Design review of the part built by this model. Coordinates are the model's own, in mm. A direction names the side the tool comes from. Coordinates: 2 decimals unless noted, no trailing zeros. Order: outer loops, then holes, each group sorted by start corner. A loop starts at its lowest first (then second) coordinate and runs counter-clockwise, first axis right, second up. Notation, with made-up numbers: (79.25, -28.75) - (86.25, -28.75) arc R20 cw to (86.25, -6.75) - close; hole circle Ø8 at (81, 15.5). An arc over 180 degrees is marked (long way). Write each question's results on one line, items separated by ' | '. Start each with the question number.
```python
from build123d import *

# Parameters (mm, degrees)
BOSS_EXTRUDE4_DEPTH = 5
SKETCH6_W           = 70
SKETCH6_H           = 70
BOSS_EXTRUDE5_DEPTH = 20
SKETCH8_R           = 3
CUT_EXTRUDE1_DEPTH  = 2
FILLET1_R           = 10
SKETCH9_W           = 24
SKETCH9_H           = 2.25
CUT_EXTRUDE2_DEPTH  = 15
SKETCH10_W          = 11.25
SKETCH10_H          = 1
CUT_EXTRUDE3_DEPTH  = 10
CHAMFER1_SIZE       = 1


with BuildPart() as part:
    # Sketch5 → Boss-Extrude4 (new body)
    with BuildSketch(Plane(origin=(0, 0, 0), x_dir=(1, 0, 0), z_dir=(0, 1, 0))):
        with BuildLine():
            Line((-22.5, -32.5), (22.5, -32.5))
            ThreePointArc((22.5, -32.5), (29.571067812, -29.571067812), (32.5, -22.5))
            Line((32.5, -22.5), (32.5, 22.5))
            ThreePointArc((32.5, 22.5), (29.571067812, 29.571067812), (22.5, 32.5))
            Line((22.5, 32.5), (-22.5, 32.5))
            ThreePointArc((-22.5, 32.5), (-29.571067812, 29.571067812), (-32.5, 22.5))
            Line((-32.5, 22.5), (-32.5, -22.5))
            ThreePointArc((-32.5, -22.5), (-29.571067812, -29.571067812), (-22.5, -32.5))
        make_face()
    extrude(amount=BOSS_EXTRUDE4_DEPTH)

    # Sketch6 → Boss-Extrude5 (add)
    with BuildSketch(Plane(origin=(0, 5, 0), x_dir=(1, 0, 0), z_dir=(0, 1, 0))):
        Rectangle(SKETCH6_W, SKETCH6_H)
    extrude(amount=BOSS_EXTRUDE5_DEPTH)

    # Sketch8 → Cut-Extrude1 (cut)
    with BuildSketch(Plane.XZ):
        with Locations(Location((26.037533906, -26.035533906, 0), (0, 0, 270))):
            Circle(SKETCH8_R)
        with Locations(Location((26.036533906, 26.036533906, 0), (0, 0, 270))):
            Circle(SKETCH8_R)
        with BuildLine():
            ThreePointArc((-23.035533906, 26.035533906), (-24.887483609, 28.807172503), (-28.156854249, 28.156854249))
            Line((-28.156854249, 28.156854249), (-23.914213562, 23.914213562))
            ThreePointArc((-23.914213562, 23.914213562), (-23.263895308, 24.887483609), (-23.035533906, 26.035533906))
        make_face()
        with BuildLine():
            Line((-23.914213562, 23.914213562), (-28.156854249, 28.156854249))
            ThreePointArc((-28.156854249, 28.156854249), (-28.156854249, 23.914213562), (-23.914213562, 23.914213562))
        make_face()
        with Locations(Location((-26.034533906, -26.036533906, 0), (0, 0, 270))):
            Circle(SKETCH8_R)
    extrude(amount=-CUT_EXTRUDE1_DEPTH, mode=Mode.SUBTRACT)

    # Fillet1
    fillet1_edges = [part.edges().sort_by_distance(p)[0] for p in [
        (-35, 15, -35),
        (-35, 15, 35),
        (35, 15, 35),
        (35, 15, -35),
    ]]
    fillet(fillet1_edges, radius=FILLET1_R)

    # Sketch9 → Cut-Extrude2 (cut)
    with BuildSketch(Plane(origin=(0, 25, 0), x_dir=(1, 0, 0), z_dir=(0, 1, 0))):
        with Locations((-13, -23.875)):
            Rectangle(SKETCH9_W, SKETCH9_H)
        with Locations((-13, -18.875)):
            Rectangle(SKETCH9_W, SKETCH9_H)
        with Locations((-13, -13.875)):
            Rectangle(SKETCH9_W, SKETCH9_H)
        with Locations((-13, -3.875)):
            Rectangle(SKETCH9_W, SKETCH9_H)
        with Locations((-13, 1.125)):
            Rectangle(SKETCH9_W, SKETCH9_H)
        with Locations((-13, 6.125)):
            Rectangle(SKETCH9_W, SKETCH9_H)
        with Locations((-13, 11.125)):
            Rectangle(SKETCH9_W, SKETCH9_H)
        with Locations((-13, 16.125)):
            Rectangle(SKETCH9_W, SKETCH9_H)
        with Locations((-13, 21.125)):
            Rectangle(SKETCH9_W, SKETCH9_H)
        with Locations((-13, -8.875)):
            Rectangle(SKETCH9_W, SKETCH9_H)
    extrude(amount=-CUT_EXTRUDE2_DEPTH, mode=Mode.SUBTRACT)

    # Sketch10 → Cut-Extrude3 (cut)
    with BuildSketch(Plane(origin=(0, 25, 0), x_dir=(1, 0, 0), z_dir=(0, 1, 0))):
        with Locations((19.375, -24.5)):
            Rectangle(SKETCH10_W, SKETCH10_H)
        with Locations((19.375, -19.5)):
            Rectangle(SKETCH10_W, SKETCH10_H)
        with Locations((19.375, -14.5)):
            Rectangle(SKETCH10_W, SKETCH10_H)
        with Locations((19.375, -9.5)):
            Rectangle(SKETCH10_W, SKETCH10_H)
        with Locations((19.375, 0.5)):
            Rectangle(SKETCH10_W, SKETCH10_H)
        with Locations((19.375, 5.5)):
            Rectangle(SKETCH10_W, SKETCH10_H)
        with Locations((19.375, 10.5)):
            Rectangle(SKETCH10_W, SKETCH10_H)
        with Locations((19.375, 15.5)):
            Rectangle(SKETCH10_W, SKETCH10_H)
        with Locations((19.375, 20.5)):
            Rectangle(SKETCH10_W, SKETCH10_H)
        with Locations((19.375, -4.5)):
            Rectangle(SKETCH10_W, SKETCH10_H)
    extrude(amount=-CUT_EXTRUDE3_DEPTH, mode=Mode.SUBTRACT)

    # Chamfer1
    chamfer1_edges = [part.edges().sort_by_distance(p)[0] for p in [
        (-25, 25, 23.875),
        (-13, 25, 22.75),
        (-13, 25, 25),
        (-1, 25, 23.875),
        (-25, 25, 8.875),
        (-13, 25, 7.75),
        (-13, 25, 10),
        (-1, 25, 8.875),
        (-13, 25, -22.25),
        (-25, 25, -21.125),
        (-13, 25, -20),
        (-1, 25, -21.125),
        (-13, 25, -17.25),
        (-25, 25, -16.125),
        (-13, 25, -15),
        (-1, 25, -16.125),
        (-13, 25, -12.25),
        (-25, 25, -11.125),
        (-13, 25, -10),
        (-1, 25, -11.125),
        (-13, 25, -7.25),
        (-25, 25, -6.125),
        (-13, 25, -5),
        (-1, 25, -6.125),
        (-13, 25, -2.25),
        (-25, 25, -1.125),
        (-13, 25, 0),
        (-1, 25, -1.125),
        (-13, 25, 2.75),
        (-25, 25, 3.875),
        (-13, 25, 5),
        (-1, 25, 3.875),
        (-13, 25, 12.75),
        (-25, 25, 13.875),
        (-13, 25, 15),
        (-1, 25, 13.875),
        (-13, 25, 17.75),
        (-25, 25, 18.875),
        (-13, 25, 20),
        (-1, 25, 18.875),
        (13.75, 25, 24.5),
        (25, 25, 24.5),
        (19.375, 25, 25),
        (19.375, 25, 24),
        (19.375, 25, 5),
        (13.75, 25, 4.5),
        (25, 25, 4.5),
        (19.375, 25, 4),
        (25, 25, -20.5),
        (19.375, 25, -20),
        (13.75, 25, -20.5),
        (19.375, 25, -21),
        (25, 25, -15.5),
        (19.375, 25, -15),
        (13.75, 25, -15.5),
        (19.375, 25, -16),
        (25, 25, -10.5),
        (19.375, 25, -10),
        (13.75, 25, -10.5),
        (19.375, 25, -11),
        (25, 25, -5.5),
        (19.375, 25, -5),
        (13.75, 25, -5.5),
        (19.375, 25, -6),
        (25, 25, -0.5),
        (19.375, 25, 0),
        (13.75, 25, -0.5),
        (19.375, 25, -1),
        (25, 25, 9.5),
        (19.375, 25, 10),
        (13.75, 25, 9.5),
        (19.375, 25, 9),
        (25, 25, 14.5),
        (19.375, 25, 15),
        (13.75, 25, 14.5),
        (19.375, 25, 14),
        (19.375, 25, 20),
        (13.75, 25, 19.5),
        (25, 25, 19.5),
        (19.375, 25, 19),
        (-35, 25, 0),
        (0, 25, -35),
        (0, 25, 35),
        (35, 25, 0),
        (32.071067812, 25, -32.071067812),
        (32.071067812, 25, 32.071067812),
        (-32.071067812, 25, 32.071067812),
        (-32.071067812, 25, -32.071067812),
    ]]
    chamfer(chamfer1_edges, length=CHAMFER1_SIZE)


solid = part.part
```
(1) Mouldability with a two-part tool opening along Z and no side actions: class faces 4 (the face through (29.65, 2.46, -29.49)), 5 (the face through (-32.15, 14.63, 31.99)), 6 (the face through (-26, 2, -26)) as +Z half, -Z half, draft (parallel to the pull), parting line (faces both ways), or undercut.
(2) Clearance check with flat-ended pins moving along their axes: pin 1 (6 mm diameter, centred on x = 20, z = 27, fed in from -Y); pin 2 (2.5 mm diameter, centred on x = -12, z = -21, fed in from +Y); pin 3 (0.5 mm diameter, centred on x = 21, z = -0.5, fed in from +Y). State where each tip first meets the part, or that it passes through.
(3) Take a section at B-B (y = 16.75). State how many separate pieces and enclosed holes the cut face has, plus the area to 3 significant figures.
(4) Tool access review of faces 1 (the face through (29.49, 2.46, 29.65)), 2 (the face through (19, 20, -21)), 3 (the face through (26, 2, 26)): name each direction out of +Z, -Z, +X, -X, +Y, -Y from which nothing blocks a thin tool from reaching the whole face with its end or side.
(5) Take a section at A-A (y = 3.25). State the section outline as (x, z) points.
Worked out:
1) face 4: -Z half | face 5: +Z half | face 6: undercut
2) pin 1: y = 0 | pin 2: y = 24.25 | pin 3: y = 15
3) separate pieces: 1 | enclosed holes: 20 | area: 4,160 mm^2
4) face 1: +Z, +X, -Y | face 2: +Y | face 3: -Y
5) outline: (-32.5, -22.5) arc R10 ccw to (-22.5, -32.5) - (22.5, -32.5) arc R10 ccw to (32.5, -22.5) - (32.5, 22.5) arc R10 ccw to (22.5, 32.5) - (-22.5, 32.5) arc R10 ccw to (-32.5, 22.5) - close
